```python
from build123d import *

# Parameters (mm, degrees)
SKETCH1_W              = 203.2
SKETCH1_H              = 152.4
BOSS_EXTRUDE1_DEPTH    = 3.175
SKETCH2_W              = 12.7
SKETCH2_H              = 3.175
BOSS_EXTRUDE2_DEPTH    = 3.175
BOSS_EXTRUDE2_2_DEPTH  = 3.175
BOSS_EXTRUDE2_3_DEPTH  = 3.175
BOSS_EXTRUDE2_4_DEPTH  = 3.175
BOSS_EXTRUDE2_5_DEPTH  = 3.175
BOSS_EXTRUDE2_6_DEPTH  = 3.175
BOSS_EXTRUDE2_7_DEPTH  = 3.175
BOSS_EXTRUDE2_8_DEPTH  = 3.175
BOSS_EXTRUDE2_9_DEPTH  = 3.175
BOSS_EXTRUDE2_10_DEPTH = 3.175
BOSS_EXTRUDE2_11_DEPTH = 3.175
BOSS_EXTRUDE2_12_DEPTH = 3.175
BOSS_EXTRUDE2_13_DEPTH = 3.175
BOSS_EXTRUDE2_14_DEPTH = 3.175
BOSS_EXTRUDE2_15_DEPTH = 3.175
BOSS_EXTRUDE2_16_DEPTH = 3.175
SKETCH4_R              = 1.375
RASPI_DEPTH            = 4.175
SKETCH5_R              = 1.6
ARDUINO_DEPTH          = 4.175
SKETCH10_R             = 1.535
SKETCH10_R_2           = 1.5
PERFBOARD_DEPTH        = 1
PERFBOARD_DEPTH_BACK   = 4.175


with BuildPart() as part:
    # Sketch1 → Boss-Extrude1 (new body)
    with BuildSketch(Plane(origin=(0, 0, 0), x_dir=(1, 0, 0), z_dir=(0, 1, 0))):
        with Locations((101.6, 76.2)):
            Rectangle(SKETCH1_W, SKETCH1_H)
    extrude(amount=BOSS_EXTRUDE1_DEPTH)

    # Sketch4 → Raspi (cut, through all)
    with BuildSketch(Plane(origin=(163.318517222, 3.175, 18.128898402), x_dir=(-1, 0, 0), z_dir=(0, 1, 0))):
        with Locations((75.468517222, -41.828898402)):
            Circle(SKETCH4_R)
        with Locations((75.468517222, -90.828898402)):
            Circle(SKETCH4_R)
        with Locations((133.468517222, -90.828898402)):
            Circle(SKETCH4_R)
        with Locations((133.468517222, -41.828898402)):
            Circle(SKETCH4_R)
    extrude(amount=-RASPI_DEPTH, mode=Mode.SUBTRACT)

    # Sketch5 → Arduino (cut, through all)
    with BuildSketch(Plane(origin=(-58.332709996, 3.175, -175.865858612), x_dir=(0, 0, 1), z_dir=(0, 1, 0))):
        with Locations((100.475405858, 205.398928035)):
            Circle(SKETCH5_R)
        with Locations((101.575405858, 253.198928035)):
            Circle(SKETCH5_R)
        with Locations((152.375405858, 210.098928035)):
            Circle(SKETCH5_R)
        with Locations((152.375405858, 237.998928035)):
            Circle(SKETCH5_R)
    extrude(amount=-ARDUINO_DEPTH, mode=Mode.SUBTRACT)

    # Sketch10 → Perfboard (cut, two sides)
    with BuildSketch(Plane(origin=(154.738240667, 3.175, -89.784200023), x_dir=(0, 0, -1), z_dir=(0, 1, 0))) as perfboard_sk:
        with Locations((-3.423776116, 144.568240667)):
            Circle(SKETCH10_R)
        with Locations((52.455799977, 144.785900219)):
            Circle(SKETCH10_R_2)
        with Locations((-3.423776116, 58.208240667)):
            Circle(SKETCH10_R)
        with Locations((52.455799977, 58.425900219)):
            Circle(SKETCH10_R_2)
    extrude(amount=PERFBOARD_DEPTH, mode=Mode.SUBTRACT)
    extrude(perfboard_sk.sketch, amount=-PERFBOARD_DEPTH_BACK, mode=Mode.SUBTRACT)


with BuildPart() as body_2:
    # Sketch2 → Boss-Extrude2 (new body)
    with BuildSketch(Plane(origin=(0, 3.175, 0), x_dir=(1, 0, 0), z_dir=(0, 1, 0))):
        with Locations((31.75, -1.5875)):
            Rectangle(SKETCH2_W, SKETCH2_H)
    extrude(amount=-BOSS_EXTRUDE2_DEPTH)


with BuildPart() as body_3:
    # Sketch2 → Boss-Extrude2 2 (new body)
    with BuildSketch(Plane(origin=(0, 3.175, 0), x_dir=(1, 0, 0), z_dir=(0, 1, 0))):
        with Locations((6.35, -1.5875)):
            Rectangle(SKETCH2_W, SKETCH2_H)
    extrude(amount=-BOSS_EXTRUDE2_2_DEPTH)


with BuildPart() as body_4:
    # Sketch2 → Boss-Extrude2 3 (new body)
    with BuildSketch(Plane(origin=(0, 3.175, 0), x_dir=(1, 0, 0), z_dir=(0, 1, 0))):
        with Locations((57.15, -1.5875)):
            Rectangle(SKETCH2_W, SKETCH2_H)
    extrude(amount=-BOSS_EXTRUDE2_3_DEPTH)


with BuildPart() as body_5:
    # Sketch2 → Boss-Extrude2 4 (new body)
    with BuildSketch(Plane(origin=(0, 3.175, 0), x_dir=(1, 0, 0), z_dir=(0, 1, 0))):
        with Locations((82.55, -1.5875)):
            Rectangle(SKETCH2_W, SKETCH2_H)
    extrude(amount=-BOSS_EXTRUDE2_4_DEPTH)


with BuildPart() as body_6:
    # Sketch2 → Boss-Extrude2 5 (new body)
    with BuildSketch(Plane(origin=(0, 3.175, 0), x_dir=(1, 0, 0), z_dir=(0, 1, 0))):
        with Locations((107.95, -1.5875)):
            Rectangle(SKETCH2_W, SKETCH2_H)
    extrude(amount=-BOSS_EXTRUDE2_5_DEPTH)


with BuildPart() as body_7:
    # Sketch2 → Boss-Extrude2 6 (new body)
    with BuildSketch(Plane(origin=(0, 3.175, 0), x_dir=(1, 0, 0), z_dir=(0, 1, 0))):
        with Locations((133.35, -1.5875)):
            Rectangle(SKETCH2_W, SKETCH2_H)
    extrude(amount=-BOSS_EXTRUDE2_6_DEPTH)


with BuildPart() as body_8:
    # Sketch2 → Boss-Extrude2 7 (new body)
    with BuildSketch(Plane(origin=(0, 3.175, 0), x_dir=(1, 0, 0), z_dir=(0, 1, 0))):
        with Locations((158.75, -1.5875)):
            Rectangle(SKETCH2_W, SKETCH2_H)
    extrude(amount=-BOSS_EXTRUDE2_7_DEPTH)


with BuildPart() as body_9:
    # Sketch2 → Boss-Extrude2 8 (new body)
    with BuildSketch(Plane(origin=(0, 3.175, 0), x_dir=(1, 0, 0), z_dir=(0, 1, 0))):
        with Locations((184.15, -1.5875)):
            Rectangle(SKETCH2_W, SKETCH2_H)
    extrude(amount=-BOSS_EXTRUDE2_8_DEPTH)


with BuildPart() as body_10:
    # Sketch2 → Boss-Extrude2 9 (new body)
    with BuildSketch(Plane(origin=(0, 3.175, 0), x_dir=(1, 0, 0), z_dir=(0, 1, 0))):
        with Locations((184.15, 153.9875)):
            Rectangle(SKETCH2_W, SKETCH2_H)
    extrude(amount=-BOSS_EXTRUDE2_9_DEPTH)


with BuildPart() as body_11:
    # Sketch2 → Boss-Extrude2 10 (new body)
    with BuildSketch(Plane(origin=(0, 3.175, 0), x_dir=(1, 0, 0), z_dir=(0, 1, 0))):
        with Locations((158.75, 153.9875)):
            Rectangle(SKETCH2_W, SKETCH2_H)
    extrude(amount=-BOSS_EXTRUDE2_10_DEPTH)


with BuildPart() as body_12:
    # Sketch2 → Boss-Extrude2 11 (new body)
    with BuildSketch(Plane(origin=(0, 3.175, 0), x_dir=(1, 0, 0), z_dir=(0, 1, 0))):
        with Locations((133.35, 153.9875)):
            Rectangle(SKETCH2_W, SKETCH2_H)
    extrude(amount=-BOSS_EXTRUDE2_11_DEPTH)


with BuildPart() as body_13:
    # Sketch2 → Boss-Extrude2 12 (new body)
    with BuildSketch(Plane(origin=(0, 3.175, 0), x_dir=(1, 0, 0), z_dir=(0, 1, 0))):
        with Locations((107.95, 153.9875)):
            Rectangle(SKETCH2_W, SKETCH2_H)
    extrude(amount=-BOSS_EXTRUDE2_12_DEPTH)


with BuildPart() as body_14:
    # Sketch2 → Boss-Extrude2 13 (new body)
    with BuildSketch(Plane(origin=(0, 3.175, 0), x_dir=(1, 0, 0), z_dir=(0, 1, 0))):
        with Locations((82.55, 153.9875)):
            Rectangle(SKETCH2_W, SKETCH2_H)
    extrude(amount=-BOSS_EXTRUDE2_13_DEPTH)


with BuildPart() as body_15:
    # Sketch2 → Boss-Extrude2 14 (new body)
    with BuildSketch(Plane(origin=(0, 3.175, 0), x_dir=(1, 0, 0), z_dir=(0, 1, 0))):
        with Locations((57.15, 153.9875)):
            Rectangle(SKETCH2_W, SKETCH2_H)
    extrude(amount=-BOSS_EXTRUDE2_14_DEPTH)


with BuildPart() as body_16:
    # Sketch2 → Boss-Extrude2 15 (new body)
    with BuildSketch(Plane(origin=(0, 3.175, 0), x_dir=(1, 0, 0), z_dir=(0, 1, 0))):
        with Locations((31.75, 153.9875)):
            Rectangle(SKETCH2_W, SKETCH2_H)
    extrude(amount=-BOSS_EXTRUDE2_15_DEPTH)


with BuildPart() as body_17:
    # Sketch2 → Boss-Extrude2 16 (new body)
    with BuildSketch(Plane(origin=(0, 3.175, 0), x_dir=(1, 0, 0), z_dir=(0, 1, 0))):
        with Locations((6.35, 153.9875)):
            Rectangle(SKETCH2_W, SKETCH2_H)
    extrude(amount=-BOSS_EXTRUDE2_16_DEPTH)


with BuildPart() as body_3_1:
    add(body_3.part)

    # Combine1: union body 4, body 6, body 8, body 10, body 12, body 14, body 16, body 17, part, body 2, body 5, body 7, body 9, body 11, body 13, body 15
    add(body_4.part)
    add(body_6.part)
    add(body_8.part)
    add(body_10.part)
    add(body_12.part)
    add(body_14.part)
    add(body_16.part)
    add(body_17.part)
    add(part.part)
    add(body_2.part)
    add(body_5.part)
    add(body_7.part)
    add(body_9.part)
    add(body_11.part)
    add(body_13.part)
    add(body_15.part)


solid = body_3_1.part
```
The model under review builds one solid part; all positions refer to its coordinate system, in mm. Round coordinates to 2 decimals unless told otherwise and drop trailing zeros. Answer in a Markdown table with one row per item.
1) For pin 1 Ø1 at (x, y) = (119, 2) entering from +Z; pin 2 Ø1.6 at (y, z) = (2.5, -154.5) entering from +X; pin 3 Ø1.6 at (x, z) = (87.85, -23.7) entering from -Y; pin 4 Ø1.6 at (x, y) = (43, 1.5) entering from -Z, all flat-tipped, find the tip position at first contact; note any pin that passes through.
Taken from the geometry:
| item | result |
|---|---|
| pin 1 | stops at z = 0 |
| pin 2 | stops at x = 190.5 |
| pin 3 | passes through |
| pin 4 | stops at z = -152.4 |
2) Consider section A-A, the plane y = 1.9. Count the separate pieces of the cut face and the enclosed holes in it, plus the area to 3 significant figures.
Taken from the geometry:
| item | result |
|---|---|
| separate pieces | 1 |
| enclosed holes | 12 |
| area | 31,500 mm² |
3) Wall thickness on line 1 along Z through (x, y) = (29.85, 1.5) (3 decimals); line 2 along X through (y, z) = (1.7, -142.24); line 3 along Z through (x, y) = (89.5, 2.9): over which ranges is each line inside the solid? List them lowest first.
Taken from the geometry:
| item | result |
|---|---|
| line 1 | z = -155.575 to -74.075, -71.325 to -25.075, -22.325 to 3.175 |
| line 2 | x = 0 to 8.45, 11.45 to 94.81, 97.81 to 203.2 |
| line 3 | z = -152.4 to 0 |
